CAD build for the part. Positions are in the model's coordinates, mm. Round coordinates to 2 decimals unless told otherwise and drop trailing zeros. Loops run counter-clockwise (first coordinate to the right, second up) from the corner with the lowest first, then second, coordinate; pieces in that order, holes last. Notation, with made-up numbers: (27.25, -19.5) -> (44.25, -19.5) arc R22 cw to (44.25, -2.5) -> close; hole circle Ø9 at (-37, -21). An arc over 180 degrees is marked (long way). Answer as CSV lines item,"result".
```python
from build123d import *

# Parameters (mm, degrees)
SKETCH1_R           = 87.5
SKETCH1_R_2         = 8.5
SKETCH1_R_3         = 61.25
BOSS_EXTRUDE1_DEPTH = 1


with BuildPart() as part:
    # Sketch1 → Boss-Extrude1 (new body)
    with BuildSketch(Plane.XY):
        Circle(SKETCH1_R)
        with Locations((0, 73.5)):
            Circle(SKETCH1_R_2, mode=Mode.SUBTRACT)
        with Locations((73.5, 0)):
            Circle(SKETCH1_R_2, mode=Mode.SUBTRACT)
        with Locations(Location((-73.5, 0, 0), (0, 0, 180))):
            Circle(SKETCH1_R_2, mode=Mode.SUBTRACT)
        with Locations(Location((0, -73.5, 0), (0, 0, 180))):
            Circle(SKETCH1_R_2, mode=Mode.SUBTRACT)
        Circle(SKETCH1_R_3, mode=Mode.SUBTRACT)
    extrude(amount=BOSS_EXTRUDE1_DEPTH)


solid = part.part
```
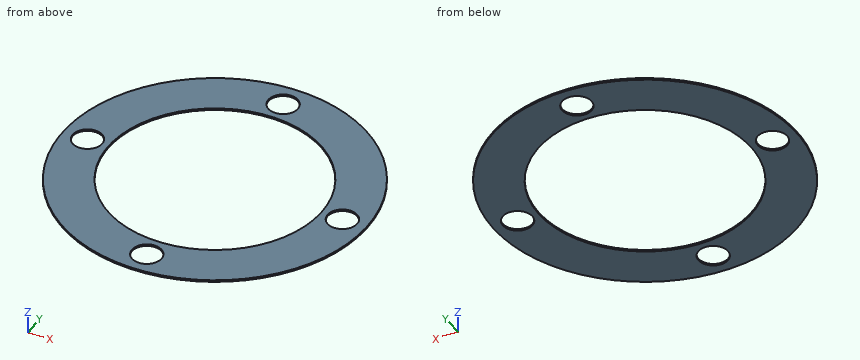
Q1. Drop a flat-ended pin along its axis: pin 1 Ø8 at (x, y) = (-47.5, -37) entering from -Z. Give the stop position or say it passes through.
Results:
pin 1,"z = 0"
Q2. Slice it at C-C, the plane x = 77.5. Give the cut face in (y, z).
Results:
outline,"(-40.62, 0) -> (-7.5, 0) -> (-7.5, 1) -> (-40.62, 1) -> close; (7.5, 0) -> (40.62, 0) -> (40.62, 1) -> (7.5, 1) -> close"
Q3. Probe L1, parallel to Y at x = 0, z = 0.7; L2, parallel to Y at x = 43.5, z = 0.55; L3, parallel to X at y = 1, z = 0.1. List the from-to ranges inside material, lowest first. Write a range as [from, to].
Results:
L1,"[-87.5, -82], [-65, -61.25], [61.25, 65], [82, 87.5]"
L2,"[-75.92, -43.12], [43.12, 75.92]"
L3,"[-87.49, -81.94], [-65.06, -61.24], [61.24, 65.06], [81.94, 87.49]"
Q4. Slice it at A-A, the plane y = 0. Give the cut face in (x, z).
Results:
outline,"(-87.5, 0) -> (-82, 0) -> (-82, 1) -> (-87.5, 1) -> close; (-65, 0) -> (-61.25, 0) -> (-61.25, 1) -> (-65, 1) -> close; (61.25, 0) -> (65, 0) -> (65, 1) -> (61.25, 1) -> close; (82, 0) -> (87.5, 0) -> (87.5, 1) -> (82, 1) -> close"
Q5. Slice it at D-D, the plane z = 0.45. Give the cut face in (x, y).
Results:
outline,"circle Ø175 at (0, 0); hole circle Ø17 at (-73.5, 0); hole circle Ø122.5 at (0, 0); hole circle Ø17 at (0, -73.5); hole circle Ø17 at (0, 73.5); hole circle Ø17 at (73.5, 0)"
